```python
from build123d import *

# Parameters (mm, degrees)
BASE_FLANGE1_DEPTH = 2028.825
SKETCH2_R          = 5.3578125
SKETCH2_R_2        = 3.429
CUT_EXTRUDE1_DEPTH = 2030.818496966
SKETCH3_R          = 3.429
SKETCH3_R_2        = 9.525
CUT_EXTRUDE2_DEPTH = 2030.880574381
FILLET1_R          = 3.175


# Sheet-metal steps are written as plain solids
with BuildPart() as part:
    # Sketch1 → Base-Flange1 (new body)
    with BuildSketch(Plane(origin=(0, 0, 0), x_dir=(0, 0, -1), z_dir=(1, 0, 0))):
        with BuildLine():
            Line((41.275, 0), (6.35, 0))
            ThreePointArc((6.35, 0), (1.859871939, -1.859871939), (0, -6.35))
            Line((0, -6.35), (0, -50.8))
            Line((0, -50.8), (3.175, -50.8))
            Line((3.175, -50.8), (3.175, -6.35))
            ThreePointArc((3.175, -6.35), (4.10493597, -4.10493597), (6.35, -3.175))
            Line((6.35, -3.175), (41.275, -3.175))
            Line((41.275, -3.175), (41.275, 0))
        make_face()
    extrude(amount=BASE_FLANGE1_DEPTH)

    # Sketch2 → Cut-Extrude1 (cut, through all)
    with BuildSketch(Plane(origin=(0, 0, -3.175), x_dir=(-1, 0, 0), z_dir=(0, 0, -1))):
        with Locations((-1873.25, -31.75)):
            Circle(SKETCH2_R)
        with Locations((-1714.5, -31.75)):
            Circle(SKETCH2_R)
        with Locations((-1695.45, -31.75)):
            Circle(SKETCH2_R)
        with Locations((-1536.7, -31.75)):
            Circle(SKETCH2_R)
        with Locations((-1206.5, -31.75)):
            Circle(SKETCH2_R)
        with Locations((-1047.75, -31.75)):
            Circle(SKETCH2_R)
        with Locations((-1028.7, -31.75)):
            Circle(SKETCH2_R)
        with Locations((-869.95, -31.75)):
            Circle(SKETCH2_R)
        with Locations((-539.75, -31.75)):
            Circle(SKETCH2_R)
        with Locations((-381, -31.75)):
            Circle(SKETCH2_R)
        with Locations((-361.95, -31.75)):
            Circle(SKETCH2_R)
        with Locations((-203.2, -31.75)):
            Circle(SKETCH2_R)
        with Locations((-9.525, -15.875)):
            Circle(SKETCH2_R_2)
        with Locations((-9.525, -34.925)):
            Circle(SKETCH2_R_2)
        with Locations((-676.275, -34.925)):
            Circle(SKETCH2_R_2)
        with Locations((-676.275, -15.875)):
            Circle(SKETCH2_R_2)
        with Locations((-1343.025, -34.925)):
            Circle(SKETCH2_R_2)
        with Locations((-1343.025, -15.875)):
            Circle(SKETCH2_R_2)
        with Locations((-2009.775, -34.925)):
            Circle(SKETCH2_R_2)
        with Locations((-2009.775, -15.875)):
            Circle(SKETCH2_R_2)
    extrude(amount=-CUT_EXTRUDE1_DEPTH, mode=Mode.SUBTRACT)

    # Sketch3 → Cut-Extrude2 (cut, through all)
    with BuildSketch(Plane(origin=(0, 0, 0), x_dir=(1, 0, 0), z_dir=(0, 1, 0))):
        with Locations(Location((2009.775, 25.4, 0), (0, 0, 270))):
            Circle(SKETCH3_R)
        with Locations(Location((1343.025, 25.4, 0), (0, 0, 270))):
            Circle(SKETCH3_R)
        with Locations(Location((676.275, 25.4, 0), (0, 0, 270))):
            Circle(SKETCH3_R)
        with Locations(Location((9.525, 25.4, 0), (0, 0, 270))):
            Circle(SKETCH3_R)
        with Locations(Location((50.8, 25.4, 0), (0, 0, 270))):
            Circle(SKETCH3_R_2)
    extrude(amount=-CUT_EXTRUDE2_DEPTH, mode=Mode.SUBTRACT)

    # Fillet1
    fillet1_edges = [part.edges().sort_by_distance(p)[0] for p in [
        (2028.825, -1.5875, -41.275),
        (0, -1.5875, -41.275),
        (2028.825, -50.8, -1.5875),
        (0, -50.8, -1.5875),
    ]]
    fillet(fillet1_edges, radius=FILLET1_R)


solid = part.part
```
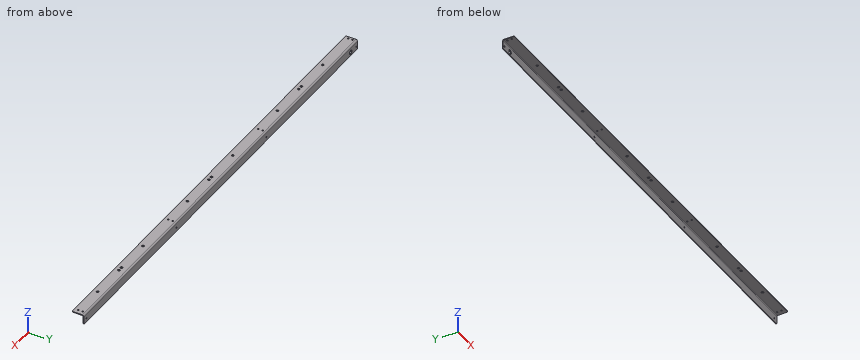
Geometry check sheet. Reference: the model listing, model coordinates, mm. Coordinates: 2 decimals unless noted, no trailing zeros. Order: outer loops, then holes, each group sorted by start corner. A loop starts at its lowest first (then second) coordinate and runs counter-clockwise, first axis right, second up. Notation, with made-up numbers: (-27.5, -4) - (7.5, -4) arc R21 cw to (7.5, 29) - close; hole circle Ø3 at (82.25, 61.5). An arc over 180 degrees is marked (long way). Answer as a JSON object with one key per item and string values. Group by question number.
Item 1: Depth check by flat-ended pin: pin 1 Ø1 at (x, y) = (280.5, -27) entering from -Z (3 decimals); pin 2 Ø2 at (x, z) = (662, -19) entering from -Y (3 decimals); pin 3 Ø1.5 at (x, y) = (979, -16.5) entering from +Z. Enter the tip coordinate at first touch or a pass-through.
Item 2: Scan lines: probe 1 along Y at (x, z) = (1695.45, -0.65); probe 2 along Z at (x, y) = (1091, -32.5) (3 decimals). Record each from-to range of solid material in increasing order.
Item 3: Sectioned sample at A-A, the plane x = 250. Record the cut outline in (y, z) (3 decimals).
Resolved:
{
 "1": {"pin 1": "z = -3.175", "pin 2": "y = -3.175", "pin 3": "z = 0"},
 "2": {"probe 1": "-50.8 to -37.11, -26.39 to -3.55", "probe 2": "-3.175 to 0"},
 "3": {"outline": "(-50.8, -3.175) - (-6.35, -3.175) arc R3.175 cw to (-3.175, -6.35) - (-3.175, -41.275) - (0, -41.275) - (0, -6.35) arc R6.35 ccw to (-6.35, 0) - (-50.8, 0) - close"}
}
